Geometry check sheet. Reference: the model listing, model coordinates, mm. A direction names the side the tool comes from. Give positions to 0.01 mm unless a question says otherwise; leave off trailing zeros. Write each loop counter-clockwise with the first axis right and the second up, starting at its lowest first coordinate (ties: lowest second). Pieces come first, ordered by that corner, then holes. Notation, with made-up numbers: (-40, 63) - (-14, 63) arc R21 cw to (-14, 90) - close; hole circle Ø5 at (21.5, 30.5). An arc over 180 degrees is marked (long way). Use a Markdown table: item, result.
```python
from build123d import *

# Parameters (mm, degrees)
BOSS_EXTRUDE1_DEPTH = 4
FILLET1_R           = 3
CUT_EXTRUDE1_DEPTH  = 5
FILLET4_R           = 3
CHAMFER1_SIZE       = 1
SKETCH3_R           = 140
CUT_EXTRUDE2_DEPTH  = 5
BOSS_EXTRUDE2_DEPTH = 5
CHAMFER2_SIZE       = 1


with BuildPart() as part:
    # Sketch1 → Boss-Extrude1 (new body)
    with BuildSketch(Plane(origin=(0, 0, 0), x_dir=(1, 0, 0), z_dir=(0, 1, 0))):
        Polygon((76, 10), (46.660254, 60.817931), (45.361216, 61.567931), (31.361216, 37.319219), (15.989265, 46.194219), (52.214265, 108.93776), (66.720191, 100.56276), (86.045101, 134.034486), (159.09982, 7.5), (120.45, 7.5), (120.45, -9.25), (48, -9.25), (48, 8.5), (76, 8.5), align=None)
    extrude(amount=BOSS_EXTRUDE1_DEPTH)

    # Fillet1
    fillet1_edges = [part.edges().sort_by_distance(p)[0] for p in [
        (48, 2, 9.25),
        (48, 2, -8.5),
        (31.361216, 2, -37.319219),
        (15.989265, 2, -46.194219),
        (52.214265, 2, -108.93776),
        (66.720191, 2, -100.56276),
        (120.45, 2, -7.5),
        (120.45, 2, 9.25),
    ]]
    fillet(fillet1_edges, radius=FILLET1_R)

    # Sketch2 → Cut-Extrude1 (cut, through all)
    with BuildSketch(Plane(origin=(0, 4, 0), x_dir=(1, 0, 0), z_dir=(0, 1, 0))):
        Polygon((46.660254, 60.817931), (45.794229, 62.317931), (45.361216, 61.567931), align=None)
        Polygon((76, 8.5), (76.866025, 8.5), (76, 10), align=None)
    extrude(amount=-CUT_EXTRUDE1_DEPTH, mode=Mode.SUBTRACT)

    # Fillet4
    fillet4_edges = [part.edges().sort_by_distance(p)[0] for p in [
        (45.794229, 2, -62.317931),
        (76.866025, 2, -8.5),
    ]]
    fillet(fillet4_edges, radius=FILLET4_R)

    # Chamfer1
    chamfer1_edges = [part.edges().sort_by_distance(p)[0] for p in [
        (61.330127, 4, -35.408965),
        (74.267949, 4, -10),
        (45.794229, 4, -59.317931),
        (23.67524, 4, -41.756719),
        (84.225, 4, 9.25),
        (120.45, 4, 0.875),
        (59.467228, 4, -104.75026),
        (34.101765, 4, -77.56599),
        (48, 4, 0.375),
        (119.57132, 4, 8.37132),
        (48.87868, 4, 8.37132),
        (48.87868, 4, -7.62132),
        (17.189564, 4, -46.515838),
        (52.535884, 4, -107.737461),
        (31.039597, 4, -38.519518),
        (66.398571, 4, -101.763059),
        (121.32868, 4, -6.62132),
    ]]
    chamfer(chamfer1_edges, length=CHAMFER1_SIZE)

    # Sketch3 → Cut-Extrude2 (cut, through all)
    with BuildSketch(Plane(origin=(0, 4, 0), x_dir=(1, 0, 0), z_dir=(0, 1, 0))):
        with Locations((226, 130.481161)):
            Circle(SKETCH3_R)
    extrude(amount=-CUT_EXTRUDE2_DEPTH, mode=Mode.SUBTRACT)

    # Sketch4 → Boss-Extrude2 (add)
    with BuildSketch(Plane.XZ):
        Polygon((20.665802, -43.494219), (56.890802, -106.23776), (62.26016, -103.13776), (26.03516, -40.394219), (23.350481, -41.944219), align=None)
        Polygon((48, 0.75), (48, 3.85), (120.45, 3.85), (120.45, -2.35), (48, -2.35), align=None)
    extrude(amount=BOSS_EXTRUDE2_DEPTH)

    # Chamfer2
    chamfer2_edges = [part.edges().sort_by_distance(p)[0] for p in [
        (84.225, -5, -2.35),
        (84.225, -5, 3.85),
        (38.778302, -5, -74.86599),
        (44.14766, -5, -71.76599),
    ]]
    chamfer(chamfer2_edges, length=CHAMFER2_SIZE)


solid = part.part
```
1) Section check A-A on x = 107.5. Record the boundary of the cut face in (y, z).
Working result:
| item | result |
|---|---|
| outline | (-5, -1.35) - (-4, -2.35) - (0, -2.35) - (0, -55.93) - (4, -55.93) - (4, 8.25) - (3, 9.25) - (0, 9.25) - (0, 3.85) - (-4, 3.85) - (-5, 2.85) - close |
2) Material ranges on L1, parallel to X at y = -3.75, z = -0.5; L2, parallel to X at y = 1.25, z = -47; L3, parallel to Z at x = 51.5, y = -1, recorded low to high. Write a range as from..to.
Working result:
| item | result |
|---|---|
| L1 | x = 48..120.45 |
| L2 | x = 17.1..36.95, 54.64..113.61 |
| L3 | z = -96.9..-84.5, -2.35..3.85 |
3) Set-up check for faces 1 (the flat face through (61.51, 1.48, -35.1)), 2 (the flat face through (85, -2, -2.35)), 3 (the flat face through (85, 0, 7)), 4 (the flat face through (83, 0, -49)): record each of +Z, -Z, +X, -X, +Y, -Y from which the full face is reachable in a straight line by a thin tool's end or side.
Working result:
| item | result |
|---|---|
| face 1 | +Y, -Y |
| face 2 | +X, -X, -Y |
| face 3 | +Z, +X, -X, -Y |
| face 4 | +X, -Y |
4) Mould release check, pull along X, two halves, no side actions. Record for faces 5 (the flat face through (38.95, -4.49, -74.18)), 6 (the flat face through (120.45, 0, 1)), 7 (the flat face through (37.674, 3.493, -49.239)): pulls with the +X half, pulls with the -X half, needs draft (parallel to the pull), parting line crosses it, or undercut.
Working result:
| item | result |
|---|---|
| face 5 | pulls with the -X half |
| face 6 | pulls with the +X half |
| face 7 | undercut |
5) Section check D-D on z = -116.5. Record the boundary of the cut face in (x, y), then the cut area to 3 significant figures.
Working result:
| item | result |
|---|---|
| outline | (75.92, 0) - (86.7, 0) - (86.7, 4) - (77.08, 4) - (75.92, 3) - close |
| area | 42.5 mm² |
6) Section check B-B on z = -91.5. Record the boundary of the cut face in (x, y), then the cut area to 3 significant figures.
Working result:
| item | result |
|---|---|
| outline | (42.15, 0) - (48.38, 0) - (48.38, -4) - (49.54, -5) - (54.39, -5) - (55.54, -4) - (55.54, 0) - (91.54, 0) - (91.54, 4) - (43.3, 4) - (42.15, 3) - close |
| area | 232 mm² |
7) Section check C-C on x = 133.5. Record the boundary of the cut face in (y, z).
Working result:
| item | result |
|---|---|
| outline | (0, -25.39) - (4, -25.39) - (4, -8.5) - (3, -7.5) - (0, -7.5) - close |
8) Depth check by flat-ended pin: P1, Ø2, axis at y = -4, z = -91, coming from the +X side; P2, Ø3, axis at y = 1.5, z = -91, coming from the -X side; P3, Ø0.9, axis at x = 142, y = 1, coming from the +Z side. Enter the tip coordinate at first touch or a pass-through.
Working result:
| item | result |
|---|---|
| P1 | stops at x = 55.83 |
| P2 | stops at x = 40.99 |
| P3 | stops at z = -7.5 |
